Geometry: final body of the model. Coordinates: model frame, mm. Give positions to 0.01 mm unless a question says otherwise; leave off trailing zeros. Write each loop counter-clockwise with the first axis right and the second up, starting at its lowest first coordinate (ties: lowest second). Pieces come first, ordered by that corner, then holes. Notation, with made-up numbers: M 82,16.25 L 110,16.25 A20 cw 110,35.25 Z; hole C -24.75,79.25 d8. An arc over 180 degrees is marked long. Use a Markdown table: item, result. Add a question column.
1) Section A-A on x = 1.5. Return the cut outline in (y, z).
2) Draft query along Y for faces 1 (the flat face through (21, 22, 1)), 2 (the cylindrical face through (41.59, 42.49, 0.49)), 3 (the flat face through (21.3, 43.25, 0.5)). Return one class per face: +Y half, -Y half, draft (parallel to the pull), parting line (faces both ways), or undercut.
3) Line query: line 1 (Y direction, x = 41.75, z = 0.35); line 2 (Y direction, x = 20, z = 0.95); line 3 (Y direction, x = 19.5, z = 0.95). Output: solid intervals per line, ascending.
4) Section B-B on z = 0.7. State how many separate pieces and enclosed holes the cut face has, then the cut area to 3 significant figures.
```python
from build123d import *

# Parameters (mm, degrees)
ESBO_O1_W                = 43.25
ESBO_O1_H                = 43.25
ESBO_O1_R                = 1.25
ESBO_O1_R_2              = 0.707384329
RESSALTO_EXTRUS_O2_DEPTH = 1


with BuildPart() as part:
    # Esboço1 → Ressalto-extrusão2 (new body)
    with BuildSketch(Plane.XY):
        with Locations((21.625, 21.625)):
            Rectangle(ESBO_O1_W, ESBO_O1_H)
        with Locations((1.5, 41.25)):
            Circle(ESBO_O1_R, mode=Mode.SUBTRACT)
        with Locations((12.322576567, 41.05)):
            Circle(ESBO_O1_R_2, mode=Mode.SUBTRACT)
        with Locations((41.75, 41.25)):
            Circle(ESBO_O1_R, mode=Mode.SUBTRACT)
        with Locations((14.892575201, 41.047350464)):
            Circle(ESBO_O1_R_2, mode=Mode.SUBTRACT)
        with Locations((17.462573835, 41.044700929)):
            Circle(ESBO_O1_R_2, mode=Mode.SUBTRACT)
        with Locations((20.03257247, 41.042051393)):
            Circle(ESBO_O1_R_2, mode=Mode.SUBTRACT)
        with Locations((22.602571104, 41.039401857)):
            Circle(ESBO_O1_R_2, mode=Mode.SUBTRACT)
        with Locations((25.172569738, 41.036752321)):
            Circle(ESBO_O1_R_2, mode=Mode.SUBTRACT)
        with Locations((27.742568372, 41.034102786)):
            Circle(ESBO_O1_R_2, mode=Mode.SUBTRACT)
        with Locations((30.312567007, 41.03145325)):
            Circle(ESBO_O1_R_2, mode=Mode.SUBTRACT)
        with Locations((30.62, 1.67673648)):
            Circle(ESBO_O1_R_2, mode=Mode.SUBTRACT)
        with Locations((28.05, 1.67673648)):
            Circle(ESBO_O1_R_2, mode=Mode.SUBTRACT)
        with Locations((25.48, 1.67673648)):
            Circle(ESBO_O1_R_2, mode=Mode.SUBTRACT)
        with Locations((22.91, 1.67673648)):
            Circle(ESBO_O1_R_2, mode=Mode.SUBTRACT)
        with Locations((20.34, 1.67673648)):
            Circle(ESBO_O1_R_2, mode=Mode.SUBTRACT)
        with Locations((17.77, 1.67673648)):
            Circle(ESBO_O1_R_2, mode=Mode.SUBTRACT)
        with Locations((15.2, 1.67673648)):
            Circle(ESBO_O1_R_2, mode=Mode.SUBTRACT)
        with Locations((41.75, 1.47673648)):
            Circle(ESBO_O1_R, mode=Mode.SUBTRACT)
        with Locations((12.63, 1.67673648)):
            Circle(ESBO_O1_R_2, mode=Mode.SUBTRACT)
        with Locations((1.5, 1.47673648)):
            Circle(ESBO_O1_R, mode=Mode.SUBTRACT)
    extrude(amount=RESSALTO_EXTRUS_O2_DEPTH)


solid = part.part
```
Found:
| question | item | result |
|---|---|---|
| 1 | outline | M 0,0 L 0.23,0 L 0.23,1 L 0,1 Z; M 2.73,0 L 40,0 L 40,1 L 2.73,1 Z; M 42.5,0 L 43.25,0 L 43.25,1 L 42.5,1 Z |
| 2 | face 1 | draft |
| 2 | face 2 | undercut |
| 2 | face 3 | +Y half |
| 3 | line 1 | 0 to 0.23, 2.73 to 40, 42.5 to 43.25 |
| 3 | line 2 | 0 to 1.06, 2.3 to 40.34, 41.75 to 43.25 |
| 3 | line 3 | 0 to 40.58, 41.51 to 43.25 |
| 4 | separate pieces | 1 |
| 4 | enclosed holes | 20 |
| 4 | area | 1,830 mm² |
